Build history of the part. All positions in model axes, mm. A direction names the side the tool comes from. Give positions to 0.01 mm unless a question says otherwise; leave off trailing zeros. Loops run counter-clockwise (first coordinate to the right, second up) from the corner with the lowest first, then second, coordinate; pieces in that order, holes last. Notation, with made-up numbers: (33.25, -38) -> (57.25, -38) arc R20 cw to (57.25, -8) -> close; hole circle Ø10 at (-15.75, -10). An arc over 180 degrees is marked (long way). Answer as a JSON object with one key per item and string values. Group by question number.
Q1. Two-plate mould, pull along Y, no slides. Class faces 1 (the flat face through (39, 42, 6)), 2 (the flat face through (39, 0, 3)), 3 (the flat face through (78, 81.5, 3)), 4 (the flat face through (15.5, 69, 3)): pulls with the +Y half, pulls with the -Y half, needs draft (parallel to the pull), parting line crosses it, or undercut.
Q2. Band-saw the part on B-B, the plane y = 5. Write the cut outline in (x, z).
Q3. Tool access for faces 5 (the flat face through (64.5, 70, 3)), 6 (the flat face through (2, 81.5, 3)): list every direction of +Z, -Z, +X, -X, +Y, -Y with a clear straight run to the whole face (end or side of a thin tool).
Q4. Band-saw the part on D-D, the plane y = 78.5. Write the cut outline in (x, z).
Q5. Wall check: probe 1 along Y at (x, z) = (40, 2.45); probe 2 along Y at (x, z) = (50.5, 2.55); probe 3 along Y at (x, z) = (20, 2.55). Give the ranges that are in metal, low to high. Write a range as from..to.
Q6. Band-saw the part on C-C, the plane x = 70. Write the cut outline in (y, z), plus the area to 3 significant figures.
Q7. Band-saw the part on A-A, the plane x = 36.5. Write the cut outline in (y, z).
Autodesk Inventor part; units mm, degrees
ref_plane "YZ Plane" through (0, 0, 0) normal (1, 0, 0) x (0, 1, 0)
ref_plane "XZ Plane" through (0, 0, 0) normal (0, 1, 0) x (-1, 0, 0)
ref_plane "XY Plane" through (0, 0, 0) normal (0, 0, 1) x (1, 0, 0)
sketch "Sketch1" plane through (0, 0, 0) normal (0, 0, 1) x (1, 0, 0)
  line L0 (4, 0) -> (76, 0)
  line L1 (80, 4) -> (80, 79.5)
  line L2 (76, 83.5) -> (4, 83.5)
  line L3 (0, 79.5) -> (0, 4)
  line L4 (0, 4) -> (4, 0)
  line L5 (76, 0) -> (80, 4)
  line L6 (80, 79.5) -> (76, 83.5)
  line L7 (4, 83.5) -> (0, 79.5)
  line L8 (16.5, 75) -> (63.5, 75)
  line L9 (64.5, 74) -> (64.5, 65)
  line L10 (63.5, 64) -> (16.5, 64)
  line L11 (15.5, 65) -> (15.5, 74)
  arc A0 (15.5, 65) -> (16.5, 64) centre (16.5, 65) ccw
  arc A1 (16.5, 75) -> (15.5, 74) centre (16.5, 74) ccw
  arc A2 (64.5, 74) -> (63.5, 75) centre (63.5, 74) ccw
  arc A3 (63.5, 64) -> (64.5, 65) centre (63.5, 65) ccw
  line L12 (28.5, 21) -> (51.5, 21)
  line L13 (52.5, 20) -> (52.5, 11)
  line L14 (51.5, 10) -> (28.5, 10)
  line L15 (27.5, 11) -> (27.5, 20)
  arc A4 (27.5, 11) -> (28.5, 10) centre (28.5, 11) ccw
  arc A5 (28.5, 21) -> (27.5, 20) centre (28.5, 20) ccw
  arc A6 (52.5, 20) -> (51.5, 21) centre (51.5, 20) ccw
  arc A7 (51.5, 10) -> (52.5, 11) centre (51.5, 11) ccw
  line L16 (15.5, 69.5) -> (64.5, 69.5) construction
  line L17 (27.5, 15.5) -> (52.5, 15.5) construction
  circle A8 centre (40, 5) radius 2.25
  circle A9 centre (10, 78.5) radius 2.25
  circle A10 centre (6, 23.25) radius 2.25
  circle A11 centre (74, 23.25) radius 2.25
  circle A12 centre (70, 78.5) radius 2.25
  point P0 (0, 0)
  point P1 (40, 64)
  point P2 (40, 21)
  point P3 (40, 75)
  point P4 (40, 83.5)
  point P5 (0, 41.75)
  point P6 (80, 41.75)
  dimension "d0" = 45
  dimension "d1" = 4
  dimension "d2" = 1
  dimension "d3" = 11
  dimension "d4" = 49
  dimension "d5" = 1
  dimension "d6" = 11
  dimension "d7" = 25
  dimension "d9" = 10
  dimension "d10" = 8.5
  dimension "d11" = 4.5
  dimension "d12" = 4.5
  dimension "d13" = 5
  dimension "d14" = 5
  dimension "d15" = 4.5
  dimension "d16" = 4.5
  dimension "d19" = 54
  dimension "d22" = 80
  dimension "d23" = 6
  dimension "d24" = 6
  dimension "d25" = 23.25
  dimension "d26" = 4.5
  dimension "d27" = 10
  dimension "d28" = 10
extrude "Extrusion2" add sketch "Sketch1" along normal blind 6
sketch "Sketch2" plane through (0, 0, 6) normal (0, 0, 1) x (1, 0, 0)
  line L0 (4, 0) -> (76, 0)
  circle A0 centre (20, 35) radius 2.25
  circle A1 centre (60, 35) radius 2.25
  line L1 (20, 35) -> (60, 35) construction
  point P0 (0, 0)
  point P1 (40, 35)
  point P2 (40, 0)
  dimension "d31" = 4.5
  dimension "d32" = 4.5
  dimension "d33" = 40
  dimension "d34" = 35
extrude "Extrusion3" cut sketch "Sketch2" against normal through all
properties part number "x_carriage"
Worked answers:
{
 "1": {"face 1": "needs draft", "face 2": "pulls with the -Y half", "face 3": "pulls with the +Y half", "face 4": "undercut"},
 "2": {"outline": "(0, 0) -> (37.75, 0) -> (37.75, 6) -> (0, 6) -> close; (42.25, 0) -> (80, 0) -> (80, 6) -> (42.25, 6) -> close"},
 "3": {"face 5": "+Z, -Z", "face 6": "+Z, -Z, -X, +Y"},
 "4": {"outline": "(0, 0) -> (7.75, 0) -> (7.75, 6) -> (0, 6) -> close; (12.25, 0) -> (67.75, 0) -> (67.75, 6) -> (12.25, 6) -> close; (72.25, 0) -> (80, 0) -> (80, 6) -> (72.25, 6) -> close"},
 "5": {"probe 1": "0..2.75, 7.25..10, 21..64, 75..83.5", "probe 2": "0..10, 21..64, 75..83.5", "probe 3": "0..32.75, 37.25..64, 75..83.5"},
 "6": {"outline": "(0, 0) -> (76.25, 0) -> (76.25, 6) -> (0, 6) -> close; (80.75, 0) -> (83.5, 0) -> (83.5, 6) -> (80.75, 6) -> close", "area": "474 mm2"},
 "7": {"outline": "(0, 0) -> (10, 0) -> (10, 6) -> (0, 6) -> close; (21, 0) -> (64, 0) -> (64, 6) -> (21, 6) -> close; (75, 0) -> (83.5, 0) -> (83.5, 6) -> (75, 6) -> close"}
}
